from build123d import *

# Parameters (mm, degrees)
SKETCH1_W               = 30
SKETCH1_H               = 55
SKETCH1_R               = 2.25
BOSS_EXTRUDE1_DEPTH     = 6
SKETCH3_W               = 30
SKETCH3_H               = 35
BOSS_EXTRUDE2_DEPTH     = 4
BOSS_EXTRUDE3_DEPTH     = 30
CUT_EXTRUDE1_DEPTH      = 52.53882032
CUT_EXTRUDE1_DEPTH_BACK = 52.53882032
SKETCH2_R               = 7.05
FILLET1_R               = 5


with BuildPart() as part:
    # Sketch1 → Boss-Extrude1 (new body)
    with BuildSketch(Plane(origin=(0, 0, 0), x_dir=(1, 0, 0), z_dir=(0, 1, 0))):
        with Locations((0, 15)):
            Rectangle(SKETCH1_W, SKETCH1_H)
        with Locations(Location((-7.5, 32.5, 0), (0, 0, 270))):
            Circle(SKETCH1_R, mode=Mode.SUBTRACT)
        with Locations(Location((7.5, 32.5, 0), (0, 0, 90))):
            Circle(SKETCH1_R, mode=Mode.SUBTRACT)
    extrude(amount=BOSS_EXTRUDE1_DEPTH)

    # Sketch3 → Boss-Extrude2 (add)
    with BuildSketch(Plane.XZ):
        with Locations((0, -5)):
            Rectangle(SKETCH3_W, SKETCH3_H)
    extrude(amount=BOSS_EXTRUDE2_DEPTH)

    # Sketch4 → Boss-Extrude3 (add)
    with BuildSketch(Plane.ZY.offset(15)):
        Polygon((-22.5, -4), (-22.5, -19), (-17.5, -19), (-7.5, -4), align=None)
    extrude(amount=-BOSS_EXTRUDE3_DEPTH)

    # Sketch2 → Cut-Extrude1 (cut, two sides: drawn at the far end of the back side and taken through both)
    with BuildSketch(Plane(origin=(0, 6, 0), x_dir=(1, 0, 0), z_dir=(0, 1, 0)).offset(-CUT_EXTRUDE1_DEPTH_BACK)):
        with Locations(Location((0, 0, 0), (0, 0, 270))):
            Circle(SKETCH2_R)
    extrude(amount=CUT_EXTRUDE1_DEPTH + CUT_EXTRUDE1_DEPTH_BACK, mode=Mode.SUBTRACT)

    # Fillet1
    fillet1_edges = [part.edges().sort_by_distance(p)[0] for p in [
        (-15, 3, -42.5),
        (15, 3, -42.5),
        (15, 1, 12.5),
        (-15, 1, 12.5),
    ]]
    fillet(fillet1_edges, radius=FILLET1_R)


solid = part.part
The model under review builds one solid part; all positions refer to its coordinate system, in mm. A direction names the side the tool comes from. Give positions to 0.01 mm unless a question says otherwise; leave off trailing zeros. Order: outer loops, then holes, each group sorted by start corner. A loop starts at its lowest first (then second) coordinate and runs counter-clockwise, first axis right, second up. Notation, with made-up numbers: M 53.25,15 L 83.25,15 A17 ccw 83.25,34 Z; hole C 58.5,65.25 d5. An arc over 180 degrees is marked long. Answer in a Markdown table with one row per item. Add a question column.
1. Mouldability with a two-part tool opening along X and no side actions: class faces 4 (the cylindrical face through (-6.824, 2.958, -30.354)), 5 (the cylindrical face through (-2.7, 0.93, 6.512)), 6 (the flat face through (0, 6, -15)), 7 (the cylindrical face through (-13.57, 3.04, -41)) as released by +X, released by -X, zero draft, split by the parting line, or undercut.
2. Machinability: for faces 1 (the flat face through (-4, -4, 7)), 2 (the flat face through (0, -9, -22.5)), 3 (the flat face through (0, 1, 12.5)), which of the approach directions +Z, -Z, +X, -X, +Y, -Y give a long, thin tool a straight path to every point of the face, cutting with its end or side? Answer none if there is none.
3. For pin 1 Ø5.5 at (x, y) = (-5.5, -6) entering from -Z; pin 2 Ø5 at (x, z) = (-10, -33.5) entering from -Y; pin 3 Ø10 at (x, z) = (-4.5, -12) entering from -Y, all flat-tipped, find the tip position at first contact; note any pin that passes through.
4. To check wall thickness, follow line 1 along X through (y, z) = (2.9, -32.5); line 2 along X through (y, z) = (-1.5, 0); line 3 along Z through (x, y) = (-0.5, -2.75). State the ranges of each line that lie inside material, in increasing order.
5. Add section A-A on z = -32.5. State the section outline as (x, y) points, plus the area to 3 significant figures.
6. Add section B-B on z = 0. State the section outline as (x, y) points, plus the area to 3 significant figures.
7. Add section D-D on x = -12.25. State the section outline as (y, z) points, plus the area to 3 significant figures.
8. Add section C-C on x = 0. State the section outline as (y, z) points, plus the area to 3 significant figures.
The answers:
| question | item | result |
|---|---|---|
| 1 | face 4 | undercut |
| 1 | face 5 | undercut |
| 1 | face 6 | zero draft |
| 1 | face 7 | released by -X |
| 2 | face 1 | +Z, +X, -X, -Y |
| 2 | face 2 | -Z, +X, -X, -Y |
| 2 | face 3 | +Z, +X, -X, +Y, -Y |
| 3 | pin 1 | z = -22.5 |
| 3 | pin 2 | y = 0 |
| 3 | pin 3 | y = -18.25 |
| 4 | line 1 | -15 to -9.75, -5.25 to 5.25, 9.75 to 15 |
| 4 | line 2 | -15 to -7.05, 7.05 to 15 |
| 4 | line 3 | -22.5 to -7.03, 7.03 to 12.5 |
| 5 | outline | M -15,0 L -9.75,0 L -9.75,6 L -15,6 Z; M -5.25,0 L 5.25,0 L 5.25,6 L -5.25,6 Z; M 9.75,0 L 15,0 L 15,6 L 9.75,6 Z |
| 5 | area | 126 mm2 |
| 6 | outline | M -15,-4 L -7.05,-4 L -7.05,6 L -15,6 Z; M 7.05,-4 L 15,-4 L 15,6 L 7.05,6 Z |
| 6 | area | 159 mm2 |
| 7 | outline | M -19,-22.5 L 0,-22.5 L 0,-41.97 L 6,-41.97 L 6,11.97 L -4,11.97 L -4,-7.5 L -19,-17.5 Z |
| 7 | area | 611 mm2 |
| 8 | outline | M -19,-22.5 L 0,-22.5 L 0,-42.5 L 6,-42.5 L 6,-7.05 L -4,-7.05 L -4,-7.5 L -19,-17.5 Z; M -4,7.05 L 6,7.05 L 6,12.5 L -4,12.5 Z |
| 8 | area | 479 mm2 |
